```python
from build123d import *

# Parameters (mm, degrees)
BASE_FLANGE1_START = -1.89738
BASE_FLANGE1_DEPTH = 1.89738
EDGE_FLANGE5_DEPTH = 1150.646018509
SKETCH21_R         = 2.778125
CUT_EXTRUDE1_DEPTH = 1.89738
SKETCH22_R         = 6.350000004
CUT_EXTRUDE2_DEPTH = 1144.944756983


# Read off the part's stored shape, not the designer's step: Base-Flange1
# Sheet-metal steps are written as plain solids
with BuildPart() as part:
    # Base-Flange1 outline → Base-Flange1 (new body)
    with BuildSketch(Plane.XY.offset(BASE_FLANGE1_START)):
        Polygon((241.231741087, -1133.16512), (441.039325341, 0), (3.468308846, 0), (3.468308846, -1133.16512), align=None)
    extrude(amount=BASE_FLANGE1_DEPTH)

    # Edge-Flange5 section (across the edge) → Edge-Flange5 (add)
    with BuildSketch(Plane(origin=(249.048652626, -1134.54345241, 0), x_dir=(-0.9848077530122076, 0.17364817766693405, 3.4914813388431337e-15), z_dir=(0.17364817766693405, 0.9848077530122076, 0))):
        with BuildLine():
            Line((-1.89738, 7.9375), (-1.89738, 48.90262))
            Line((-1.89738, 48.90262), (0, 48.90262))
            Line((0, 48.90262), (0, 7.9375))
            ThreePointArc((0, 7.9375), (2.324839924, 2.324839924), (7.9375, 0))
            Line((7.9375, 0), (7.9375, -1.89738))
            ThreePointArc((7.9375, -1.89738), (0.98318966, 0.98318966), (-1.89738, 7.9375))
        make_face()
    extrude(amount=EDGE_FLANGE5_DEPTH)

    # Sketch21 → Cut-Extrude1 (cut)
    with BuildSketch(Plane.XY):
        with Locations((416.722567093, -21.43125)):
            Circle(SKETCH21_R)
        with Locations((226.222567093, -21.43125)):
            Circle(SKETCH21_R)
        with Locations((61.122567093, -21.43125)):
            Circle(SKETCH21_R)
        with Locations((24.899558846, -200.266935)):
            Circle(SKETCH21_R)
        with Locations((24.899558846, -581.266935)):
            Circle(SKETCH21_R)
        with Locations((24.899558846, -962.266935)):
            Circle(SKETCH21_R)
    extrude(amount=-CUT_EXTRUDE1_DEPTH, mode=Mode.SUBTRACT)

    # Sketch22 → Cut-Extrude2 (cut, through all)
    with BuildSketch(Plane(origin=(435.557273959, -76.800499043, 0), x_dir=(0, 0, 1), z_dir=(-0.9848077530122062, 0.17364817766694032, 3.3536738181639377e-15))):
        with Locations(Location((28.26512, 25.785675125, 0), (0, 0, 270))):
            Circle(SKETCH22_R)
        with Locations(Location((28.26512, -327.287334129, 0), (0, 0, 270))):
            Circle(SKETCH22_R)
        with Locations(Location((28.26512, -670.187334129, 0), (0, 0, 270))):
            Circle(SKETCH22_R)
        with Locations(Location((28.26512, -1023.260343384, 0), (0, 0, 270))):
            Circle(SKETCH22_R)
    extrude(amount=-CUT_EXTRUDE2_DEPTH, mode=Mode.SUBTRACT)


solid = part.part
```
Part model, mm, in its own coordinate system. A direction names the side the tool comes from. Round coordinates to 2 decimals unless told otherwise and drop trailing zeros. Order: outer loops, then holes, each group sorted by start corner. A loop starts at its lowest first (then second) coordinate and runs counter-clockwise, first axis right, second up. Notation, with made-up numbers: M 0,56.25 L 9,56.25 A21 cw 9,66.25 Z; hole C 65.5,32 d9. An arc over 180 degrees is marked long. Answer in a Markdown table with one row per item. Add a question column.
Q1. Pin check, flat tips, straight feed: pin 1 (8 mm diameter, centred on x = 87, y = -855, fed in from +Z); pin 2 (4 mm diameter, centred on y = -193, z = 12.5, fed in from -X); pin 3 (3.5 mm diameter, centred on x = 24.9, y = -962.27, fed in from -Z); pin 4 (1 mm diameter, centred on y = -295.5, z = 28, fed in from -X). Stop position of each tip, or through.
Q2. Mould opens along Z. For faces 3 (the face through (349.422, -576.223, 28.133)), 4 (the face through (345.325, -575.5, 2.387)), 5 (the face through (171, -559, -1.897)) say: +Z half, -Z half, draft (parallel to the pull), parting line (faces both ways), or undercut.
Q3. Wall check: L1, parallel to Z at x = 208.5, y = -516; L2, parallel to Z at x = 327, y = -655; L3, parallel to X at y = -706.5, z = 35.5. Give the ranges that are in metal, low to high. Write a range as from..to.
Q4. Cut at A-A on x = 156.5. Give the cut face in (y, z), and give its area (3 significant figures).
Q5. 3-axis set-ups, long thin cutter, end or side, ignore diameter. For faces 1 (the face through (349, -576, 48.903)), 2 (the face through (171, -559, 0)): which of +Z, -Z, +X, -X, +Y, -Y reach the whole face in a straight line?
Established:
| question | item | result |
|---|---|---|
| 1 | pin 1 | stops at z = 0 |
| 1 | pin 2 | stops at x = 414.72 |
| 1 | pin 3 | passes through |
| 1 | pin 4 | stops at x = 396.91 |
| 2 | face 3 | draft |
| 2 | face 4 | +Z half |
| 2 | face 5 | -Z half |
| 3 | L1 | z = -1.9..0 |
| 3 | L2 | z = -1.79..0.13 |
| 3 | L3 | x = 324.52..326.45 |
| 4 | outline | M -1133.17,-1.9 L 0,-1.9 L 0,0 L -1133.17,0 Z |
| 4 | area | 2,150 mm2 |
| 5 | face 1 | +Z, +X, -X, +Y, -Y |
| 5 | face 2 | +Z, -X, +Y |
